```python
from build123d import *

# Parameters (mm, degrees)
F0_R     = 16.623406
F1_DEPTH = 127
F0_R_2   = 59.47353
F2_DEPTH = 76.2
F3_DEPTH = 76.2


with BuildPart() as f1:
    # F0 (on Top) → F1 (new body)
    with BuildSketch(Plane.XY):
        with Locations((81.678741, 89.352399)):
            Circle(F0_R)
    extrude(amount=F1_DEPTH)

    # F0 (on Top) → F2 (join)
    with BuildSketch(Plane.XY):
        with Locations((63.5, 109.985226)):
            Circle(F0_R_2)
        with Locations((81.678741, 89.352399)):
            Circle(F0_R, mode=Mode.SUBTRACT)
    extrude(amount=F2_DEPTH)

    # F0 (on Top) → F3 (join)
    with BuildSketch(Plane.XY):
        with BuildLine():
            ThreePointArc((127, 0), (63.5, 236.985226), (0, 0))
            Line((0, 0), (127, 0))
        make_face()
        with Locations((63.5, 109.985226)):
            Circle(F0_R_2, mode=Mode.SUBTRACT)
    extrude(amount=F3_DEPTH)


solid = f1.part
```
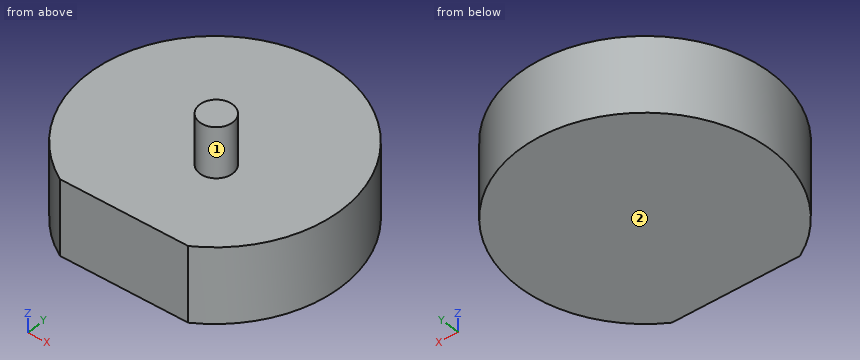
Design review of the part built by this model. Coordinates are the model's own, in mm. Face numbers are marked on the shaded views. A direction names the side the tool comes from. Coordinates: 2 decimals unless noted, no trailing zeros. Order: outer loops, then holes, each group sorted by start corner. A loop starts at its lowest first (then second) coordinate and runs counter-clockwise, first axis right, second up.
1) Take a section at A-A, the plane x = 77. Give the boundary of the cut face in (y, z).
2) Clearance check with flat-ended pins moving along their axes: pin 1 (10 mm diameter, centred on x = 82, y = 85, fed in from -Z); pin 2 (1 mm diameter, centred on x = 76.5, z = 45, fed in from +Y); pin 3 (3 mm diameter, centred on x = 80.5, z = 48, fed in from +Y). State where each tip first meets the part, or that it passes through.
3) For the marked faces 1 and 2, list the 3-axis set-ups (+Z, -Z, +X, -X, +Y, -Y) from which the entire face can be reached by the end or side of a thin tool; tool diameter is ignored.
4) Take a section at B-B, the plane z = 44. Give the boundary of the cut face in (x, y), and give its area (3 significant figures).
5) Wall thickness on line 1 along Z through (x, y) = (71, 65); line 2 along Y through (x, z) = (159, 53); line 3 along X through (y, z) = (128, 32): over which ranges is each line inside the solid? List them lowest first.
6) Take a section at C-C, the plane y = 180.5. Give the boundary of the cut face in (x, z), and give its area (3 significant figures).
7) Take a section at D-D, the plane z = 97. Give the boundary of the cut face in (x, y), and give its area (3 significant figures).
Returned:
1. outline: (0, 0) - (236.27, 0) - (236.27, 76.2) - (105.3, 76.2) - (105.3, 127) - (73.4, 127) - (73.4, 76.2) - (0, 76.2) - close
2. pin 1: stops at z = 0
2. pin 2: stops at y = 236.37
2. pin 3: stops at y = 236.04
3. face 1: +Z
3. face 2: -Z, +X, -X, +Y, -Y
4. outline: (0, 0) - (127, 0) arc R127 ccw (long way) to start
4. area: 49,200 mm2
5. line 1: z = 0 to 76.2
5. line 2: y = 26.27 to 193.7
5. line 3: x = -62.22 to 189.22
6. outline: (-42.13, 0) - (169.13, 0) - (169.13, 76.2) - (-42.13, 76.2) - close
6. area: 16,100 mm2
7. outline: circle Ø33.25 at (81.68, 89.35)
7. area: 868 mm2
